Input: part model. Units: mm. Frame: model coordinates. Face numbers are marked on the shaded views. A direction names the side the tool comes from. Give positions to 0.01 mm unless a question says otherwise; leave off trailing zeros. Loops run counter-clockwise (first coordinate to the right, second up) from the corner with the lowest first, then second, coordinate; pieces in that order, holes last. Notation, with made-up numbers: M 28,57 L 81,57 A21 cw 81,80 Z; hole C -12,52 d4. An arc over 180 degrees is marked long. Use CSV: the item, a comma, the result in double quotes. Start each with the question number.
Q1. Reachability of the marked faces 4 and 5 from +Z, -Z, +X, -X, +Y, -Y: full face, straight path, thin tool, end or side. Return the list, or none.
Q2. Pin query (flat end, axial travel): pin 1 (1.5 mm diameter, centred on x = -2, y = 119.5, fed in from +Z); pin 2 (5 mm diameter, centred on x = 14, y = 186, fed in from -Z); pin 3 (2 mm diameter, centred on x = 225.5, z = -34, fed in from -Y). Return the tip coordinate at first contact, or that it passes through.
Q3. Section A-A, the plane z = 0. Output: boundary loops of the cut face in (x, y), plus the area to 3 significant figures.
Q4. Section B-B, the plane x = 168. Output: boundary loops of the cut face in (y, z).
Q5. Pull-direction query (Y, two-part tool) for the marked faces 1, 2 and 3; classes: released by +Y, released by -Y, zero draft, split by the parting line, or undercut.
Q6. Material intervals for line 1 along Z through (x, y) = (188, 304.8); line 2 along X through (y, z) = (155, 35); line 3 along Y through (x, z) = (175, 36), sorted ascending.
from build123d import *

# Parameters (mm, degrees)
F0_R     = 76.2
F3_T     = -25.4
F0_R_2   = 95.25
F4_DEPTH = 25.4
F6_R     = 95.25
F6_R_2   = 76.2
F7_DEPTH = 25.4


with BuildPart() as f2:
    # F2: sweep along a path in F1
    with BuildLine(Plane.XY) as f2_path:
        Line((0, 0), (0, 152.4))
        ThreePointArc((0, 152.4), (44.6369265472, 260.1630734528), (152.4, 304.8))
        Line((152.4, 304.8), (304.8, 304.8))
    # F0 (on Front) → F2 (sweep)
    with BuildSketch(Plane.XZ):
        Circle(F0_R)
    sweep(path=f2_path.line)

    # F3
    f3_openings = [f2.faces().sort_by_distance(p)[0] for p in [
        (0, 0, 0),
        (304.8, 304.8, 0),
    ]]
    offset(amount=F3_T, openings=f3_openings)

    # F0 (on Front) → F4 (join)
    with BuildSketch(Plane.XZ):
        Circle(F0_R_2)
        Circle(F0_R, mode=Mode.SUBTRACT)
    extrude(amount=-F4_DEPTH)

    # F6 (on line) → F7 (join)
    with BuildSketch(Plane.YZ.offset(304.8)):
        with Locations((304.8, 0)):
            Circle(F6_R)
        with Locations((304.8, 0)):
            Circle(F6_R_2, mode=Mode.SUBTRACT)
    extrude(amount=-F7_DEPTH)


solid = f2.part
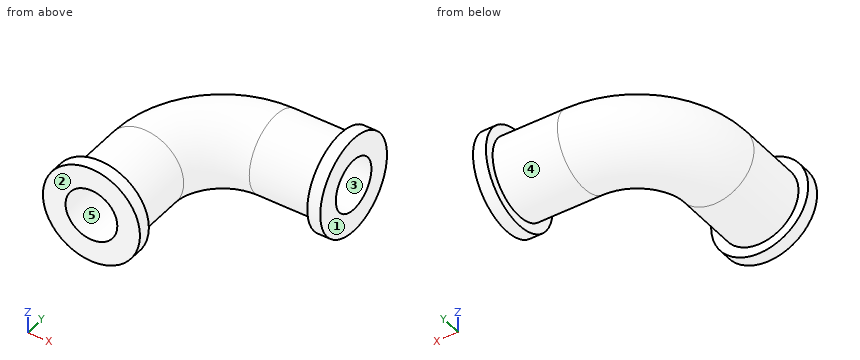
A:
1,face 4,"none"
1,face 5,"-Y"
2,pin 1,"z = 76.19"
2,pin 2,"z = -75.83"
2,pin 3,"y = 236.12"
3,outline,"M -95.25,0 L -50.8,0 L -50.8,152.4 A203.2 cw 152.4,355.6 L 304.8,355.6 L 304.8,400.05 L 279.4,400.05 L 279.4,381 L 152.4,381 A228.6 ccw -76.2,152.4 L -76.2,25.4 L -95.25,25.4 Z; M 50.8,0 L 95.25,0 L 95.25,25.4 L 76.2,25.4 L 76.2,152.4 A76.2 cw 152.4,228.6 L 279.4,228.6 L 279.4,209.55 L 304.8,209.55 L 304.8,254 L 152.4,254 A101.6 ccw 50.8,152.4 Z"
3,area,"29,600 mm^2"
4,outline,"C 304.8,0 d152.4; hole C 304.8,0 d101.6"
5,face 1,"zero draft"
5,face 2,"released by -Y"
5,face 3,"undercut"
6,line 1,"-76.2 to -50.8, 50.8 to 76.2"
6,line 2,"-67.67 to -36.8, 36.85 to 67.73"
6,line 3,"237.64 to 268.96, 340.64 to 371.96"
